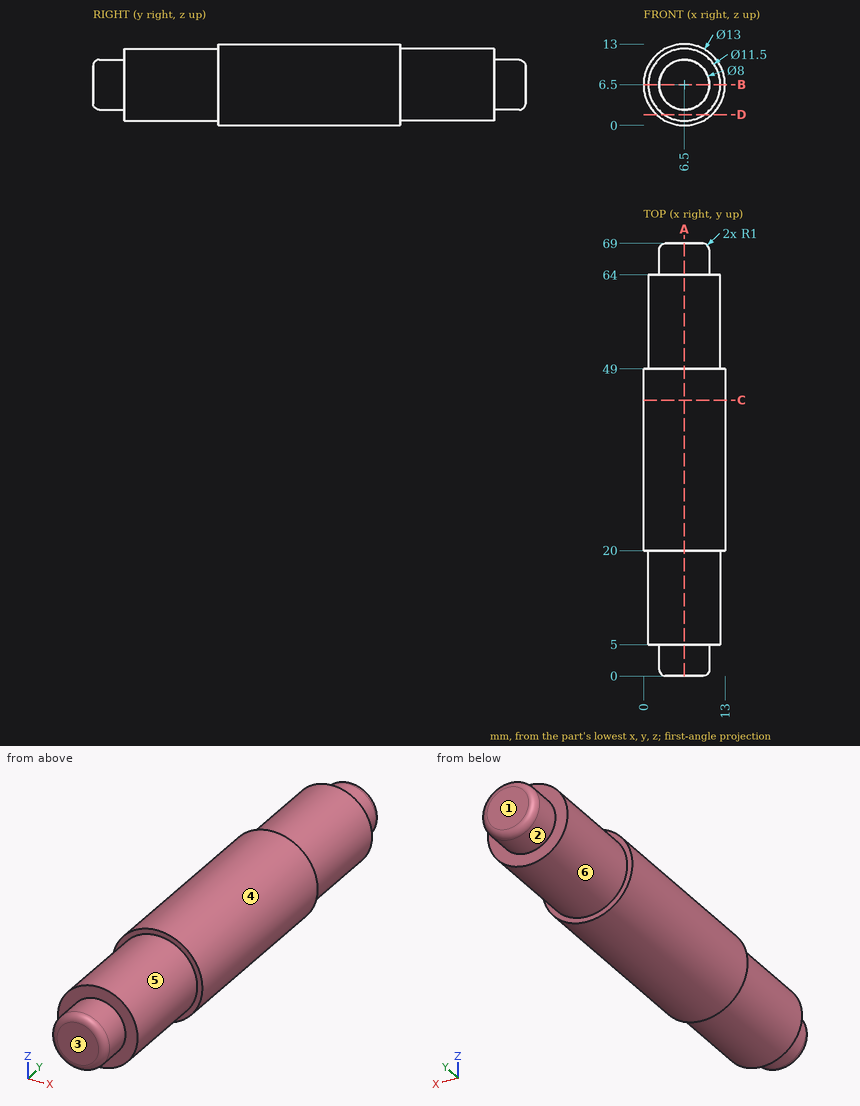
Design review of the part shown in the three views and the two pictorial views. Dimensions are in mm from the part's minimum x, y and z. A direction names the side the tool comes from. Coordinates: 2 decimals unless noted, no trailing zeros. Write each loop counter-clockwise with the first axis right and the second up, starting at its lowest first coordinate (ties: lowest second). Pieces come first, ordered by that corner, then holes.
(1) For pin 1 Ø6 at (x, y) = (10, 23.5) entering from -Z; pin 2 Ø1 at (x, z) = (4, 9.5) entering from -Y; pin 3 Ø4 at (y, z) = (15.5, 3.5) entering from +X, all flat-tipped, find the tip position at first contact; note any pin that passes through.
(2) The part is to be moulded in two halves that separate along Y. For the marked faces 1, 2 and 3, say which applies: +Y half, -Y half, draft (parallel to the pull), parting line (faces both ways), or undercut.
(3) Add section D-D on z = 1.75. Give the boundary of the cut face in (x, y).
(4) Wall thickness on probe 1 along Y at (x, z) = (7.75, 11); probe 2 along Y at (x, z) = (9.75, 11.75); probe 3 along Z at (x, y) = (6.5, 51.5): over which ranges is each line inside the solid? List them lowest first.
(5) Tool access review of the marked faces 4, 5 and 6: name each direction out of +Z, -Z, +X, -X, +Y, -Y from which nothing blocks a thin tool from reaching the whole face with its end or side.
(6) Add section B-B on z = 6.5. Give the boundary of the cut face in (x, y), then the cut area to 3 significant figures.
(7) Add section C-C on y = 44. Give the boundary of the cut face in (x, z), then the cut area to 3 significant figures.
(8) Add section A-A on x = 6.5. Give the boundary of the cut face in (y, z).
Answer sheet:
1. pin 1: stops at z = 0.02
1. pin 2: stops at y = 0.09
1. pin 3: stops at x = 12.16
2. face 1: +Y half
2. face 2: draft
2. face 3: -Y half
3. outline: (2.06, 20) - (3.26, 20) - (3.26, 5) - (9.74, 5) - (9.74, 20) - (10.94, 20) - (10.94, 49) - (9.74, 49) - (9.74, 64) - (3.26, 64) - (3.26, 49) - (2.06, 49) - close
4. probe 1: y = 5 to 64
4. probe 2: y = 20 to 49
4. probe 3: z = 0.75 to 12.25
5. face 4: +Y, -Y
5. face 5: -Y
5. face 6: +Y
6. outline: (0, 20) - (0.75, 20) - (0.75, 5) - (2.5, 5) - (2.5, 1) arc R1 ccw to (3.5, 0) - (9.5, 0) arc R1 ccw to (10.5, 1) - (10.5, 5) - (12.25, 5) - (12.25, 20) - (13, 20) - (13, 49) - (12.25, 49) - (12.25, 64) - (10.5, 64) - (10.5, 68) arc R1 ccw to (9.5, 69) - (3.5, 69) arc R1 ccw to (2.5, 68) - (2.5, 64) - (0.75, 64) - (0.75, 49) - (0, 49) - close
6. area: 801 mm2
7. outline: circle Ø13 at (6.5, 6.5)
7. area: 133 mm2
8. outline: (0, 3.5) arc R1 ccw to (1, 2.5) - (5, 2.5) - (5, 0.75) - (20, 0.75) - (20, 0) - (49, 0) - (49, 0.75) - (64, 0.75) - (64, 2.5) - (68, 2.5) arc R1 ccw to (69, 3.5) - (69, 9.5) arc R1 ccw to (68, 10.5) - (64, 10.5) - (64, 12.25) - (49, 12.25) - (49, 13) - (20, 13) - (20, 12.25) - (5, 12.25) - (5, 10.5) - (1, 10.5) arc R1 ccw to (0, 9.5) - close
